```python
from build123d import *

# Parameters (mm, degrees)
SKETCH1_W               = 42
SKETCH1_H               = 42
BOSS_EXTRUDE1_DEPTH     = 9.4
CHAMFER1_SIZE           = 5
BOSS_EXTRUDE3_DEPTH     = 21.2
BOSS_EXTRUDE6_DEPTH     = 9.4
SKETCH6_W               = 16
SKETCH6_H               = 4
BOSS_EXTRUDE7_DEPTH     = 4.4
SKETCH7_W               = 16.005281852
SKETCH7_H               = 4.99851403
SKETCH7_W_2             = 15.005281852
SKETCH7_H_2             = 3.99851403
BOSS_EXTRUDE8_DEPTH     = 6.5
CUT_EXTRUDE1_DEPTH      = 0.5
SKETCH9_W               = 1.5
SKETCH9_H               = 1
BOSS_EXTRUDE9_DEPTH     = 6
SKETCH10_R              = 11
BOSS_EXTRUDE10_DEPTH    = 2
SKETCH11_R              = 2.5
BOSS_EXTRUDE11_DEPTH    = 18
CUT_EXTRUDE3_DEPTH      = 70.262183044
CUT_EXTRUDE3_DEPTH_BACK = 16
CUT_EXTRUDE4_START      = -0.5
SKETCH13_R              = 14
SKETCH13_R_2            = 11
CUT_EXTRUDE4_DEPTH      = 0.5
CIRPATTERN2_COUNT       = 4
CHAMFER3_SIZE           = 0.5
FILLET1_R               = 1
CHAMFER4_SIZE           = 0.5


with BuildPart() as part:
    # Sketch1 → Boss-Extrude1 (new body)
    with BuildSketch(Plane.XY):
        Rectangle(SKETCH1_W, SKETCH1_H)
    extrude(amount=BOSS_EXTRUDE1_DEPTH)

    # Chamfer1
    chamfer1_edges = [part.edges().sort_by_distance(p)[0] for p in [
        (-21, 21, 4.7),
        (21, 21, 4.7),
        (21, -21, 4.7),
        (-21, -21, 4.7),
    ]]
    chamfer(chamfer1_edges, length=CHAMFER1_SIZE)

    # Sketch3 → Boss-Extrude3 (add)
    with BuildSketch(Plane.XY.offset(9.4)):
        Polygon((-12, 21), (-21, 12), (-21, -12), (-12, -21), (12, -21), (21, -12), (21, 12), (12, 21), align=None)
    extrude(amount=BOSS_EXTRUDE3_DEPTH)

    # Sketch5 → Boss-Extrude6 (add)
    with BuildSketch(Plane.XY.offset(30.6)):
        Polygon((21, 12), (12, 21), (-12, 21), (-21, 12), (-21, -12), (-12, -21), (12, -21), (21, -12), align=None)
        Polygon((-12, 21), (-16, 21), (-21, 16), (-21, 12), align=None)
        Polygon((16, 21), (12, 21), (21, 12), (21, 16), align=None)
        Polygon((21, -16), (21, -12), (12, -21), (16, -21), align=None)
        Polygon((-12, -21), (-21, -12), (-21, -16), (-16, -21), align=None)
    extrude(amount=BOSS_EXTRUDE6_DEPTH)

    # Sketch6 → Boss-Extrude7 (add)
    with BuildSketch(Plane(origin=(0, 0, 0), x_dir=(-1, 0, 0), z_dir=(0, 0, -1))):
        with Locations((-0.000479461, 23)):
            Rectangle(SKETCH6_W, SKETCH6_H)
    extrude(amount=-BOSS_EXTRUDE7_DEPTH)

    # Sketch7 → Boss-Extrude8 (add)
    with BuildSketch(Plane(origin=(0, 21, 0), x_dir=(1, 0, 0), z_dir=(0, 1, 0))):
        with Locations((0.003120387, -6.899257015)):
            Rectangle(SKETCH7_W, SKETCH7_H)
        with Locations((0.003120387, -6.899257015)):
            Rectangle(SKETCH7_W_2, SKETCH7_H_2, mode=Mode.SUBTRACT)
    extrude(amount=BOSS_EXTRUDE8_DEPTH)

    # Sketch8 → Cut-Extrude1 (cut)
    with BuildSketch(Plane.XY.offset(9.39851403)):
        Polygon((-5.999520539, 25.5), (-5.999520539, 29.381183142), (6.005761313, 29.381183142), (6.005761313, 25.5), (6.005761313, 23), (-5.999520539, 23), align=None)
    extrude(amount=-CUT_EXTRUDE1_DEPTH, mode=Mode.SUBTRACT)

    # Sketch9 → Boss-Extrude9 (add)
    with BuildSketch(Plane(origin=(0, 21, 0), x_dir=(1, 0, 0), z_dir=(0, 1, 0))):
        with Locations((-5.149520539, -6.8)):
            Rectangle(SKETCH9_W, SKETCH9_H)
        with Locations((-1.649520539, -6.8)):
            Rectangle(SKETCH9_W, SKETCH9_H)
        with Locations((1.850479461, -6.8)):
            Rectangle(SKETCH9_W, SKETCH9_H)
        with Locations((5.350479461, -6.8)):
            Rectangle(SKETCH9_W, SKETCH9_H)
    extrude(amount=BOSS_EXTRUDE9_DEPTH)

    # Sketch10 → Boss-Extrude10 (add)
    with BuildSketch(Plane.XY.offset(40)):
        Circle(SKETCH10_R)
    extrude(amount=BOSS_EXTRUDE10_DEPTH)

    # Sketch11 → Boss-Extrude11 (add)
    with BuildSketch(Plane.XY.offset(42)):
        Circle(SKETCH11_R)
    extrude(amount=BOSS_EXTRUDE11_DEPTH)

    # Sketch12 → Cut-Extrude3 (cut, two sides: drawn at the far end of the back side and taken through both)
    with BuildSketch(Plane.XY.offset(60).offset(-CUT_EXTRUDE3_DEPTH_BACK)):
        Polygon((-81.426219831, 1.5), (-2, 1.5), (2, 1.5), (81.426219831, 1.5), (81.426219831, 160.352439662), (-81.426219831, 160.352439662), align=None)
    extrude(amount=CUT_EXTRUDE3_DEPTH + CUT_EXTRUDE3_DEPTH_BACK, mode=Mode.SUBTRACT)

    # Sketch13 → Cut-Extrude4 (cut)
    with BuildSketch(Plane.XY.offset(40).offset(CUT_EXTRUDE4_START)):
        Circle(SKETCH13_R)
        Circle(SKETCH13_R_2, mode=Mode.SUBTRACT)
    extrude(amount=CUT_EXTRUDE4_DEPTH, mode=Mode.SUBTRACT)

    # Sketch15 → #4-40 Tapped Hole1 (revolve, cut)
    with BuildSketch(Plane(origin=(-15.5, 15.5, 40), x_dir=(0, -1, 0), z_dir=(1, 0, 0))):
        Polygon((0, 0), (0, 9.179152758), (1.1303, 8.5), (1.1303, 0.9271), (2.0574, 0), align=None)
    f_4_40_tapped_hole1 = revolve(axis=Axis((-15.5, 15.5, 46.35), (0, 0, -1)), mode=Mode.SUBTRACT)

    # CirPattern2: #4-40 Tapped Hole1 ×4 about axis
    cirpattern2_axis = Axis((0, 0, 0), (0, 0, 1))
    for i in range(1, CIRPATTERN2_COUNT):
        add(f_4_40_tapped_hole1.rotate(cirpattern2_axis, i * 360 / CIRPATTERN2_COUNT), mode=Mode.SUBTRACT)

    # Chamfer3
    chamfer3_edges = [part.edges().sort_by_distance(p)[0] for p in [
        (-11, 0, 42),
        (-2.5, 0, 42),
        (-0.790569415, -2.371708245, 60),
        (0, 2.5, 44),
        (-14, 0, 40),
    ]]
    chamfer(chamfer3_edges, length=CHAMFER3_SIZE - 0.0001)  # a hair under: the kernel refuses the full size

    # Fillet1
    fillet1_edges = [part.edges().sort_by_distance(p)[0] for p in [
        (21, 16, 4.7),
        (21, -16, 4.7),
        (-16, -21, 4.7),
        (16, -21, 4.7),
        (-21, 16, 4.7),
        (-21, -16, 4.7),
        (16, 21, 4.7),
        (-16, 21, 4.7),
        (12, 21, 20),
        (-12, 21, 20),
        (-21, 12, 20),
        (-21, -12, 20),
        (-12, -21, 20),
        (12, -21, 20),
        (21, -12, 20),
        (21, 12, 20),
        (21, -16, 35.3),
        (21, 16, 35.3),
        (16, 21, 35.3),
        (-16, 21, 35.3),
        (-21, 16, 35.3),
        (-21, -16, 35.3),
        (-16, -21, 35.3),
        (16, -21, 35.3),
    ]]
    fillet(fillet1_edges, radius=FILLET1_R)

    # Chamfer4
    chamfer4_edges = [part.edges().sort_by_distance(p)[0] for p in [
        (-11.792653488, 21, 0),
        (8.000479461, 25, 2.2),
        (-7.999520539, 25, 2.2),
        (8.000479461, 23, 0),
        (0.000479461, 25, 0),
        (0, 21, 40),
        (11.79313295, 21, 0),
        (-18.5, 18.5, 0),
        (21, 0, 0),
        (18.5, -18.5, 0),
        (0, -21, 0),
        (-18.5, -18.5, 0),
        (-21, 0, 0),
        (18.5, 18.5, 0),
        (20.923879533, 15.96846987, 0),
        (15.96846987, 20.923879533, 0),
        (20.923879533, -15.96846987, 0),
        (15.96846987, -20.923879533, 0),
        (-15.96846987, -20.923879533, 0),
        (-20.923879533, -15.96846987, 0),
        (-20.923879533, 15.96846987, 0),
        (-15.96846987, 20.923879533, 0),
        (-18.5, 18.5, 40),
        (21, 0, 40),
        (18.5, 18.5, 40),
        (-21, 0, 40),
        (-18.5, -18.5, 40),
        (0, -21, 40),
        (18.5, -18.5, 40),
        (15.96846987, 20.923879533, 40),
        (20.923879533, 15.96846987, 40),
        (20.923879533, -15.96846987, 40),
        (15.96846987, -20.923879533, 40),
        (-15.96846987, -20.923879533, 40),
        (-20.923879533, -15.96846987, 40),
        (-20.923879533, 15.96846987, 40),
        (-15.96846987, 20.923879533, 40),
    ]]
    chamfer(chamfer4_edges, length=CHAMFER4_SIZE)


solid = part.part
```
For this review, take the finished solid that the model builds, in its own axes (mm). A direction names the side the tool comes from. Round coordinates to 2 decimals unless told otherwise and drop trailing zeros. Write each loop counter-clockwise with the first axis right and the second up, starting at its lowest first coordinate (ties: lowest second). Pieces come first, ordered by that corner, then holes. Notation, with made-up numbers: (82, -8.5) -> (136, -8.5) arc R30 cw to (136, 23.5) -> close; hole circle Ø8 at (7, 31.25). An arc over 180 degrees is marked (long way). One line per question, with ' | ' between items. Start each with the question number.
(1) Mouldability with a two-part tool opening along Y and no side actions: class faces 4 (the face through (14.397, -15.745, 35.339)), 5 (the face through (-17, 17, 9.4)), 6 (the face through (-18.29, 18.36, 39.75)), 7 (the face through (-15.51, 15.7, 30.94)) as released by +Y, released by -Y, zero draft, split by the parting line, or undercut.
(2) Add section A-A, the plane z = 36.5. Write out the cut boundary in (x, y).
(3) For line 1 along Y through (x, z) = (-15.5, 37); line 2 along Y through (x, z) = (-15, 33), list the stretches that pass through material, from the lowest coordinate up. Write a range as from..to.
(4) Tool access review of faces 1 (the face through (-7.5, 24, 7)), 2 (the face through (17, 16, 20)), 3 (the face through (-17, -18, 9.4)): name each direction out of +Z, -Z, +X, -X, +Y, -Y from which nothing blocks a thin tool from reaching the whole face with its end or side.
(5) Add section C-C, the plane z = 11.5. Write out the cut boundary in (x, y).
(6) Insertion check: P1, Ø4, axis at y = 25.5, z = 7, coming from the +X side; P2, Ø12, axis at x = -1, y = -7, coming from the +Z side; P3, Ø0.8, axis at x = -2, y = 25, coming from the -Z side; P4, Ø0.8, axis at x = 5, z = 7, coming from the +Y side. Each pin has a flat end and moves straight along its axis. Give the tip position at first contact, or say it passes through.
(7) Add section D-D, the plane z = 53. Write out the cut boundary in (x, y).
Answer list:
1) face 4: undercut | face 5: zero draft | face 6: released by +Y | face 7: undercut
2) outline: (-21, -15.59) arc R1 ccw to (-20.71, -16.29) -> (-16.29, -20.71) arc R1 ccw to (-15.59, -21) -> (15.59, -21) arc R1 ccw to (16.29, -20.71) -> (20.71, -16.29) arc R1 ccw to (21, -15.59) -> (21, 15.59) arc R1 ccw to (20.71, 16.29) -> (16.29, 20.71) arc R1 ccw to (15.59, 21) -> (-15.59, 21) arc R1 ccw to (-16.29, 20.71) -> (-20.71, 16.29) arc R1 ccw to (-21, 15.59) -> close; hole circle Ø2.26 at (-15.5, -15.5); hole circle Ø2.26 at (-15.5, 15.5); hole circle Ø2.26 at (15.5, -15.5); hole circle Ø2.26 at (15.5, 15.5)
3) line 1: -21..-16.63, -14.37..14.37, 16.63..21 | line 2: -21..-16.51, -14.49..14.49, 16.51..21
4) face 1: +Y | face 2: +X, +Y | face 3: -X, -Y
5) outline: (-21, -11.59) arc R1 ccw to (-20.71, -12.29) -> (-12.29, -20.71) arc R1 ccw to (-11.59, -21) -> (11.59, -21) arc R1 ccw to (12.29, -20.71) -> (20.71, -12.29) arc R1 ccw to (21, -11.59) -> (21, 11.59) arc R1 ccw to (20.71, 12.29) -> (12.29, 20.71) arc R1 ccw to (11.59, 21) -> (-11.59, 21) arc R1 ccw to (-12.29, 20.71) -> (-20.71, 12.29) arc R1 ccw to (-21, 11.59) -> close
6) P1: x = 8.01 | P2: z = 60 | P3: z = 0.1 | P4: y = 27
7) outline: (-2, 1.5) arc R2.5 ccw (long way) to (2, 1.5) -> close
